Part model, mm, in its own coordinate system. A direction names the side the tool comes from. Give positions to 0.01 mm unless a question says otherwise; leave off trailing zeros. Order: outer loops, then holes, each group sorted by start corner. A loop starts at its lowest first (then second) coordinate and runs counter-clockwise, first axis right, second up. Notation, with made-up numbers: (-8.5, 4) -> (29.5, 4) arc R7 ccw to (29.5, 17) -> close; hole circle Ø4 at (21, 49). An arc over 180 degrees is marked (long way). Write item = value, one per line. Start each with the question number.
Item 1: Band-saw the part on C-C on x = -55. Write the cut outline in (y, z), plus the area to 4 significant figures.
Item 2: Band-saw the part on D-D on x = 55. Write the cut outline in (y, z).
Item 3: Flat gauge pins, fed straight in: P1, Ø0.6, axis at y = 3.5, z = 7, coming from the +X side; P2, Ø1, axis at y = -24, z = 7, coming from the -X side; P3, Ø1, axis at x = -36, z = 7, coming from the +Y side. Where does each tip first touch, or does it go through?
Item 4: Tool access for faces 1 (the face through (-15, 58, 4)), 2 (the face through (100, -2, 3)): list every direction of +Z, -Z, +X, -X, +Y, -Y with a clear straight run to the whole face (end or side of a thin tool).
Item 5: Drill centre lines: line 1 along X through (y, z) = (57, 5); line 2 along X through (y, z) = (-11.5, 7.25); line 3 along Z through (x, y) = (44.5, 53). Where is each one in solid material? Low to high.
Item 6: Band-saw the part on A-A on x = 18. Write the cut outline in (y, z).
Item 7: Band-saw the part on B-B on y = -33.5. Write the cut outline in (x, z), plus the area to 3 significant figures.
```python
from build123d import *

# Parameters (mm, degrees)
SKETCH_W        = 200
SKETCH_H        = 125
PAD_DEPTH       = 6
SKETCH001_W     = 177
SKETCH001_H     = 102
PAD001_DEPTH    = 2
POCKET_DEPTH    = 120
SKETCH003_W     = 85
SKETCH003_H     = 10
POCKET001_DEPTH = 8.001
FILLET_R        = 2
CHAMFER_SIZE    = 1
CHAMFER001_SIZE = 1
CHAMFER002_SIZE = 1


with BuildPart() as part:
    # Sketch → Pad (new body)
    with BuildSketch(Plane.XY):
        Rectangle(SKETCH_W, SKETCH_H)
    extrude(amount=PAD_DEPTH)

    # Sketch001 (on Face6 of Pad) → Pad001 (join)
    with BuildSketch(Plane.XY.offset(6)):
        Rectangle(SKETCH001_W, SKETCH001_H)
    extrude(amount=PAD001_DEPTH)

    # Sketch002 (on Face2 of Pad001) → Pocket (cut)
    with BuildSketch(Plane(origin=(-100, 0, 0), x_dir=(0, -1, 0), z_dir=(-1, 0, 0))):
        Polygon((-60.5, 0), (-56.964466, 3.535534), (-53.428932, 0), (-56.964466, -3.535534), align=None)
    extrude(amount=-POCKET_DEPTH, mode=Mode.SUBTRACT)

    # Sketch003 (on Face4 of Pocket) → Pocket001 (cut, through all)
    with BuildSketch(Plane(origin=(0, 0, 0), x_dir=(1, 0, 0), z_dir=(0, 0, -1))):
        with Locations((-57.5, -57.5)):
            Rectangle(SKETCH003_W, SKETCH003_H)
    extrude(amount=-POCKET001_DEPTH, mode=Mode.SUBTRACT)

    # Fillet
    fillet_edges = [part.edges().sort_by_distance(p)[0] for p in [
        (100, 62.5, 3),
    ]]
    fillet(fillet_edges, radius=FILLET_R)

    # Chamfer
    chamfer_edges = [part.edges().sort_by_distance(p)[0] for p in [
        (100, -1, 0),
    ]]
    chamfer(chamfer_edges, length=CHAMFER_SIZE)

    # Chamfer001
    chamfer001_edges = [part.edges().sort_by_distance(p)[0] for p in [
        (-100, -5, 0),
    ]]
    chamfer(chamfer001_edges, length=CHAMFER001_SIZE)

    # Chamfer002
    chamfer002_edges = [part.edges().sort_by_distance(p)[0] for p in [
        (0, -62.5, 0),
    ]]
    chamfer(chamfer002_edges, length=CHAMFER002_SIZE)


solid = part.part
```
Values found:
q1.outline = (-62.5, 1) -> (-61.5, 0) -> (52.5, 0) -> (52.5, 6) -> (51, 6) -> (51, 8) -> (-51, 8) -> (-51, 6) -> (-62.5, 6) -> close
q1.area = 893.5 mm^2
q2.outline = (-62.5, 1) -> (-61.5, 0) -> (61.5, 0) -> (62.5, 1) -> (62.5, 6) -> (51, 6) -> (51, 8) -> (-51, 8) -> (-51, 6) -> (-62.5, 6) -> close
q3.P1 = 88.5
q3.P2 = -88.5
q3.P3 = 51
q4.face_1 = +Z, -Z, -X, +Y
q4.face_2 = +Z, -Z, +X, +Y, -Y
q5.line_1 = -15 to 100
q5.line_2 = -88.5 to 88.5
q5.line_3 = 0 to 6
q6.outline = (-62.5, 1) -> (-61.5, 0) -> (53.43, 0) -> (56.96, 3.54) -> (60.5, 0) -> (61.5, 0) -> (62.5, 1) -> (62.5, 6) -> (51, 6) -> (51, 8) -> (-51, 8) -> (-51, 6) -> (-62.5, 6) -> close
q7.outline = (-100, 1) -> (-99, 0) -> (99, 0) -> (100, 1) -> (100, 6) -> (88.5, 6) -> (88.5, 8) -> (-88.5, 8) -> (-88.5, 6) -> (-100, 6) -> close
q7.area = 1,550 mm^2
